Autodesk Fusion 360 part; units mm, degrees
sketch "Sketch1" plane through (0, 0, 0) normal (0, 0, 1) x (1, 0, 0)
  line L0 (0, 6.35) -> (0, 0)
  line L1 (0, 0) -> (76.2, 0)
  line L2 (76.2, 0) -> (76.2, 31.75)
  line L3 (76.2, 31.75) -> (0, 88.9)
  line L4 (0, 88.9) -> (0, 82.55)
  line L5 (0, 82.55) -> (-20.828, 82.55)
  line L6 (-20.828, 82.55) -> (-20.828, 6.35)
  line L7 (-20.828, 6.35) -> (0, 6.35)
  line L8 (10, 0) -> (10, 130)
  line L9 (-221.1749, 94.6346) -> (-221.1749, -30.5637)
  line L10 (10, 130) -> (98.9697, -9.6544)
  line L11 (98.9697, -9.6544) -> (98.9697, -74.6544)
  line L12 (98.9697, -74.6544) -> (10, 0)
  dimension "d1" = 10
  dimension "d12" = 130
  dimension "d15" = 32.5
  dimension "d18" = 130
  dimension "d22" = 65
extrude "Extrude1" add sketch "Sketch1" along normal blind 3.175 contours L1 L2 L3 L8 L10 | L1 L2 L10 L11 L12 | L3 L8 L10 makes body 1
copy_body "Body->Comp1" bodies 1 removing the originals makes body 2 in component "Component"
sketch "Sketch3" plane through (10, 0, 0) normal (-1, 0, 0) x (0, 0, 1)
  line L0 (0, 130) -> (0, 0)
  line L1 (0, 0) -> (3.175, 0)
  line L2 (3.175, 0) -> (3.175, 130)
  line L3 (0, 12.7) -> (3.175, 12.7)
  line L4 (0, 88.9) -> (3.175, 88.9)
  line L5 (3.175, 130) -> (0, 130)
  dimension "d20" = 12.7
  dimension "d21" = 76.2
extrude "Extrude1'" add sketch "Sketch3" along normal blind 12.7 contours L0 L2 L3 L4 bodies 2 in component "Component"
component "Component" placed x (1, 0, 0) y (0, 1, 0) z (0, 0, 1) at (0, 0, 0)
equation "d2 = ( 1 / 8 ) * 1 in"
Can you work these out from the model? Positions are in its coordinate system, mm. Give positions to 0.01 mm unless a question says otherwise; leave off trailing zeros. Loops run counter-clockwise (first coordinate to the right, second up) from the corner with the lowest first, then second, coordinate; pieces in that order, holes last. Notation, with made-up numbers: M 49.25,-12 L 102.25,-12 A23 cw 102.25,16 Z; hole C 49.5,50.5 d4. An arc over 180 degrees is marked long. Answer in a Markdown table with one row per item.
1. Suppose I cut it at A-A on z = 1.1. Write out the boundary of the cut face in (x, y).
Taken from the geometry:
| item | result |
|---|---|
| outline | M -2.7,12.7 L 10,12.7 L 10,0 L 98.97,-74.65 L 98.97,-9.65 L 10,130 L 10,88.9 L -2.7,88.9 Z |
2. Suppose I cut it at B-B on y = -22. Write out the boundary of the cut face in (x, z) (3 decimals).
Taken from the geometry:
| item | result |
|---|---|
| outline | M 36.219,0 L 98.97,0 L 98.97,3.175 L 36.219,3.175 Z |
3. Suppose I cut it at C-C on x = 13. Write out the boundary of the cut face in (y, z) (3 decimals).
Taken from the geometry:
| item | result |
|---|---|
| outline | M -2.517,0 L 125.291,0 L 125.291,3.175 L -2.517,3.175 Z |
4. For pin 1 Ø1 at (x, z) = (43, 1) entering from +Y; pin 2 Ø1.5 at (x, z) = (58, 2) entering from -Y; pin 3 Ø1 at (y, z) = (5.5, 1.5) entering from -X, each with a flat end and sliding along its axis, tell me the tip position at first contact or that it passes through.
Taken from the geometry:
| item | result |
|---|---|
| pin 1 | stops at y = 78.99 |
| pin 2 | stops at y = -40.91 |
| pin 3 | stops at x = 10 |
5. If I drill on line 1 along Y through (x, z) = (93, 1.9); line 2 along Y through (x, z) = (67, 2.3); line 3 along X through (y, z) = (18, 0.4), over which ranges is the centre line in solid material (lowest first)?
Taken from the geometry:
| item | result |
|---|---|
| line 1 | y = -69.65 to -0.28 |
| line 2 | y = -47.83 to 40.53 |
| line 3 | x = -2.7 to 81.35 |
